from build123d import *

# Parameters (mm, degrees)
F1_DEPTH = 6.35
F2_START = 50.8
F2_DEPTH = 6.35
F3_DEPTH = 57.15


with BuildPart() as f1:
    # F0 (on Right) → F1 (new body)
    with BuildSketch(Plane.YZ):
        with BuildLine():
            Line((-49.3914086659, -58.3716647869), (-0.7353354825, -9.7155916035))
            ThreePointArc((-0.7353354825, -9.7155916035), (-3.7417609774, -8.2639811349), (-5.3244428604, -5.3244428604))
            Line((-5.3244428604, -5.3244428604), (-53.8815367264, -53.8815367264))
            Line((-53.8815367264, -53.8815367264), (-49.3914086659, -58.3716647869))
        make_face()
    extrude(amount=F1_DEPTH)



with BuildPart() as f1b:
    # F0 (on Right) → F1, piece 2 (new body)
    with BuildSketch(Plane.YZ):
        with BuildLine():
            Line((53.8815367264, -53.8815367264), (5.3244428604, -5.3244428604))
            ThreePointArc((5.3244428604, -5.3244428604), (3.7417609774, -8.2639811349), (0.7353354825, -9.7155916035))
            Line((0.7353354825, -9.7155916035), (49.3914086659, -58.3716647869))
            Line((49.3914086659, -58.3716647869), (53.8815367264, -53.8815367264))
        make_face()
    extrude(amount=F1_DEPTH)


with BuildPart() as f2:
    # F0 (on Right) → F2 (new body)
    with BuildSketch(Plane.YZ.offset(F2_START)):
        with BuildLine():
            Line((-49.3914086659, -58.3716647869), (-0.7353354825, -9.7155916035))
            ThreePointArc((-0.7353354825, -9.7155916035), (-3.7417609774, -8.2639811349), (-5.3244428604, -5.3244428604))
            Line((-5.3244428604, -5.3244428604), (-53.8815367264, -53.8815367264))
            Line((-53.8815367264, -53.8815367264), (-49.3914086659, -58.3716647869))
        make_face()
    extrude(amount=F2_DEPTH)


with BuildPart() as f2b:
    # F0 (on Right) → F2, piece 2 (new body)
    with BuildSketch(Plane.YZ.offset(F2_START)):
        with BuildLine():
            Line((53.8815367264, -53.8815367264), (5.3244428604, -5.3244428604))
            ThreePointArc((5.3244428604, -5.3244428604), (3.7417609774, -8.2639811349), (0.7353354825, -9.7155916035))
            Line((0.7353354825, -9.7155916035), (49.3914086659, -58.3716647869))
            Line((49.3914086659, -58.3716647869), (53.8815367264, -53.8815367264))
        make_face()
    extrude(amount=F2_DEPTH)


with BuildPart() as f1_1:
    add(f1.part)

    add(f1b.part)  # F3 merges F1b

    add(f2.part)  # F3 merges F2

    add(f2b.part)  # F3 merges F2b
    # F0 (on Right) → F3 (join)
    with BuildSketch(Plane.YZ):
        with BuildLine():
            ThreePointArc((0.7353354825, -9.7155916035), (3.7417609774, -8.2639811349), (5.3244428604, -5.3244428604))
            ThreePointArc((5.3244428604, -5.3244428604), (5.3902466222, -4.8409706351), (5.4122407959, -4.3535367586))
            ThreePointArc((5.4122407959, -4.3535367586), (-0.4874338766, 1.0367098636), (-5.3244428604, -5.3244428604))
            ThreePointArc((-5.3244428604, -5.3244428604), (-3.7417609774, -8.2639811349), (-0.7353354825, -9.7155916035))
            ThreePointArc((-0.7353354825, -9.7155916035), (0, -9.7657775544), (0.7353354825, -9.7155916035))
        make_face()
    extrude(amount=F3_DEPTH)


solid = f1_1.part
Verification items for the finished model (mm, model axes). A direction names the side the tool comes from. Give positions to 0.01 mm unless a question says otherwise; leave off trailing zeros. Loops run counter-clockwise (first coordinate to the right, second up) from the corner with the lowest first, then second, coordinate; pieces in that order, holes last. Notation, with made-up numbers: (59, -28) - (98, -28) arc R16 ccw to (98, -6) - close; hole circle Ø4 at (54, -16.5). An arc over 180 degrees is marked (long way). Write item = value, one per line. Start each with the question number.
Q1. Cross-section at C-C, the plane y = -33.5. Enter the section's corners in (x, z).
Q2. Depth check by flat-ended pin: P1, Ø3, axis at x = 12.5, y = -3, coming from the -Z side; P2, Ø4, axis at x = 14.5, z = -7, coming from the +Y side; P3, Ø8, axis at x = 49.5, z = -38.5, coming from the -Y side. Enter the tip coordinate at first touch or a pass-through.
Q3. Cross-section at B-B, the plane z = -39.5. Enter the section's corners in (x, y).
Q4. Cross-section at A-A, the plane x = 46. Enter the section's corners in (y, z).
Q5. Thickness scan on line 1 (X direction, y = -28, z = -35); line 2 (Y direction, x = 53.5, z = -37); line 3 (Z direction, x = 51.5, y = -41). Record the ranges inside material, lowest first.
Q6. Mould release check, pull along X, two halves, no side actions. Record for faces 1 (the face through (50.8, 27, -34)), 2 (the face through (3, -29, -29)), 3 (the face through (6.35, 27, -34)), 4 (the face through (57.15, -12, -20)): released by +X, released by -X, zero draft, split by the parting line, or undercut.
Q7. Tool access check on faces 5 (the face through (53.93, -25.4, -34.38)), 6 (the face through (53.931, -51.668, -56.095)). Record the directions out of +Z, -Z, +X, -X, +Y, -Y that give a thin tool (end or side, any length) a straight path to the whole face; none if there is none.
Answer key:
q1.outline = (0, -42.48) - (6.35, -42.48) - (6.35, -33.5) - (0, -33.5) - close; (50.8, -42.48) - (57.15, -42.48) - (57.15, -33.5) - (50.8, -33.5) - close
q2.P1 = -9.55
q2.P2 = 5.37
q2.P3 = -42.28
q3.outline = (0, -39.5) - (6.35, -39.5) - (6.35, -30.52) - (0, -30.52) - close; (0, 30.52) - (6.35, 30.52) - (6.35, 39.5) - (0, 39.5) - close; (50.8, -39.5) - (57.15, -39.5) - (57.15, -30.52) - (50.8, -30.52) - close; (50.8, 30.52) - (57.15, 30.52) - (57.15, 39.5) - (50.8, 39.5) - close
q4.outline = circle Ø10.82 at (0, -4.35)
q5.line_1 = 0 to 6.35, 50.8 to 57.15
q5.line_2 = -37 to -28.02, 28.02 to 37
q5.line_3 = -49.98 to -41
q6.face_1 = undercut
q6.face_2 = zero draft
q6.face_3 = undercut
q6.face_4 = released by +X
q7.face_5 = -Z, +X, -X
q7.face_6 = -Z, +X, -X, -Y
